Design review of the part built by this model. Coordinates are the model's own, in mm. A direction names the side the tool comes from. Round coordinates to 2 decimals unless told otherwise and drop trailing zeros. Order: outer loops, then holes, each group sorted by start corner. A loop starts at its lowest first (then second) coordinate and runs counter-clockwise, first axis right, second up. Notation, with made-up numbers: (36.25, 50.5) - (55.25, 50.5) arc R29 ccw to (55.25, 89.5) - close; hole circle Ø7 at (47.5, -36). An arc over 180 degrees is marked (long way). Use CSV: the item, a comma, the result in double quotes.
from build123d import *

# Parameters (mm, degrees)
SKETCH1_W               = 12.04
SKETCH1_H               = 7.58
SKETCH1_W_2             = 8.04
SKETCH1_H_2             = 3.58
BOSS_EXTRUDE1_DEPTH     = 8
SKETCH1_2_W             = 12.04
SKETCH1_2_H             = 7.58
SKETCH1_2_W_2           = 8.04
SKETCH1_2_H_2           = 3.58
BOSS_EXTRUDE2_DEPTH     = 2
CHAMFER1_SIZE           = 1.5
CUT_EXTRUDE1_DEPTH      = 13.55773865
CUT_EXTRUDE1_DEPTH_BACK = 13.55773865
FILLET1_R               = 0.5
CHAMFER2_SIZE           = 1


with BuildPart() as part:
    # Sketch1 → Boss-Extrude1 (new body)
    with BuildSketch(Plane.XY):
        Rectangle(SKETCH1_W, SKETCH1_H)
        Rectangle(SKETCH1_W_2, SKETCH1_H_2, mode=Mode.SUBTRACT)
    extrude(amount=BOSS_EXTRUDE1_DEPTH)

    # Sketch1_2 → Boss-Extrude2 (add)
    # profile 1 of 2: a face of its own
    with BuildSketch(Plane.XY):
        Rectangle(SKETCH1_2_W, SKETCH1_2_H)
        Rectangle(SKETCH1_2_W_2, SKETCH1_2_H_2, mode=Mode.SUBTRACT)
    # profile 2 of 2: a face of its own
    with BuildSketch(Plane.XY):
        Rectangle(SKETCH1_2_W_2, SKETCH1_2_H_2)
    extrude(amount=-BOSS_EXTRUDE2_DEPTH)

    # Chamfer1
    chamfer1_edges = [part.edges().sort_by_distance(p)[0] for p in [
        (6.02, -3.79, 3),
        (-6.02, -3.79, 3),
        (-6.02, 3.79, 3),
        (6.02, 3.79, 3),
    ]]
    chamfer(chamfer1_edges, length=CHAMFER1_SIZE)

    # Sketch2 → Cut-Extrude1 (cut, two sides: drawn at the far end of the back side and taken through both)
    with BuildSketch(Plane.XZ.offset(3.79).offset(-CUT_EXTRUDE1_DEPTH_BACK)):
        Polygon((-1.905255888, 2.9), (1.905255888, 2.9), (0, 6.2), align=None)
    extrude(amount=CUT_EXTRUDE1_DEPTH + CUT_EXTRUDE1_DEPTH_BACK, mode=Mode.SUBTRACT)

    # Fillet1
    fillet1_edges = [part.edges().sort_by_distance(p)[0] for p in [
        (-1.905255888, -2.79, 2.9),
        (0, -2.79, 6.2),
        (1.905255888, -2.79, 2.9),
        (-1.905255888, 2.79, 2.9),
        (0, 2.79, 6.2),
        (1.905255888, 2.79, 2.9),
    ]]
    fillet(fillet1_edges, radius=FILLET1_R)

    # Chamfer2
    chamfer2_edges = [part.edges().sort_by_distance(p)[0] for p in [
        (0, -3.79, -2),
        (6.02, 0, -2),
        (-6.02, 0, -2),
        (0, 3.79, -2),
        (5.27, -3.04, -2),
        (5.27, 3.04, -2),
        (-5.27, 3.04, -2),
        (-5.27, -3.04, -2),
    ]]
    chamfer(chamfer2_edges, length=CHAMFER2_SIZE)


solid = part.part
1) To check wall thickness, follow L1, parallel to X at y = -0.5, z = 3.25; L2, parallel to Y at x = 2.5, z = 6.75; L3, parallel to Z at x = -0.5, y = 0.75. State the ranges of each line that lie inside material, in increasing order. Write a range as from..to.
Data:
L1,"x = -6.02..-4.02, 4.02..6.02"
L2,"y = -3.79..-1.79, 1.79..3.79"
L3,"z = -2..0"
2) We need section A-A (z = 5.25). Give the boundary of the cut face in (x, y), then the cut area to 3 significant figures.
Data:
outline,"(-6.02, -2.29) - (-4.52, -3.79) - (-0.55, -3.79) - (-0.55, -1.79) - (-4.02, -1.79) - (-4.02, 1.79) - (-0.55, 1.79) - (-0.55, 3.79) - (-4.52, 3.79) - (-6.02, 2.29) - close; (0.55, -3.79) - (4.52, -3.79) - (6.02, -2.29) - (6.02, 2.29) - (4.52, 3.79) - (0.55, 3.79) - (0.55, 1.79) - (4.02, 1.79) - (4.02, -1.79) - (0.55, -1.79) - close"
area,"53.6 mm2"
3) The part is to be moulded in two halves that separate along Y. For faces 4 (the face through (-6.02, 0, 4)), 5 (the face through (4.02, 0, 4)), 6 (the face through (-0.1, 3.79, 2.6)), say which applies: +Y half, -Y half, draft (parallel to the pull), parting line (faces both ways), or undercut.
Data:
face 4,"draft"
face 5,"undercut"
face 6,"+Y half"
4) We need section C-C (z = 2.75). Give the boundary of the cut face in (x, y), then the cut area to 3 significant figures.
Data:
outline,"(-6.02, -2.29) - (-4.52, -3.79) - (4.52, -3.79) - (6.02, -2.29) - (6.02, 2.29) - (4.52, 3.79) - (-4.52, 3.79) - (-6.02, 2.29) - close; hole (-4.02, -1.79) - (4.02, -1.79) - (4.02, 1.79) - (-4.02, 1.79) - close"
area,"58.0 mm2"
5) We need section B-B (x = -3.75). Give the boundary of the cut face in (y, z), then the cut area to 3 significant figures.
Data:
outline,"(-3.79, -1) - (-2.79, -2) - (2.79, -2) - (3.79, -1) - (3.79, 8) - (1.79, 8) - (1.79, 0) - (-1.79, 0) - (-1.79, 8) - (-3.79, 8) - close"
area,"46.2 mm2"
6) Insertion check: pin 1 Ø1.1 at (x, y) = (0.5, -0.5) entering from +Z. The pin has a flat end and moves straight along its axis. Give the tip position at first contact, or say it passes through.
Data:
pin 1,"stops at z = 0"
7) For faces 1 (the face through (-1, -1.79, 5)), 2 (the face through (0, 2.8, 5.7)), 3 (the face through (-0.06, 3.3, -1.49)), list the 3-axis set-ups (+Z, -Z, +X, -X, +Y, -Y) from which the entire face can be reached by the end or side of a thin tool; tool diameter is ignored.
Data:
face 1,"+Z"
face 2,"+Y, -Y"
face 3,"-Z, +X, -X, +Y"
8) We need section D-D (y = 1.25). Give the boundary of the cut face in (x, z).
Data:
outline,"(-6.02, -1) - (-5.02, -2) - (5.02, -2) - (6.02, -1) - (6.02, 8) - (4.02, 8) - (4.02, 0) - (-4.02, 0) - (-4.02, 8) - (-6.02, 8) - close"
